```python
from build123d import *

# Parameters (mm, degrees)
SKETCH_1_R      = 1.55
SKETCH_1_W      = 16
SKETCH_1_H      = 6
EXTRUDE_1_DEPTH = 2.2
CHAMFER_1_SIZE  = 3


with BuildPart() as part:
    # 草图1 → 凸台-拉伸1 (new body)
    with BuildSketch(Plane(origin=(0, 0, 0), x_dir=(0, 0, -1), z_dir=(1, 0, 0))):
        with BuildLine():
            Line((-14, -11.5), (14, -11.5))
            Line((14, -11.5), (14, -7.01))
            ThreePointArc((14, -7.01), (12.995, -6.005), (14, -5))
            Line((14, -5), (17, -5))
            Line((17, -5), (17, 5))
            Line((17, 5), (14, 5))
            ThreePointArc((14, 5), (12.995, 6.005), (14, 7.01))
            Line((14, 7.01), (14, 11.5))
            Line((14, 11.5), (6.01, 11.5))
            ThreePointArc((6.01, 11.5), (5.005, 10.495), (4, 11.5))
            Line((4, 11.5), (4, 13.7))
            Line((4, 13.7), (-4, 13.7))
            Line((-4, 13.7), (-4, 11.5))
            ThreePointArc((-4, 11.5), (-5.005, 10.495), (-6.01, 11.5))
            Line((-6.01, 11.5), (-14, 11.5))
            Line((-14, 11.5), (-14, 7.01))
            ThreePointArc((-14, 7.01), (-13.289357685, 6.715642315), (-12.995, 6.005))
            ThreePointArc((-12.995, 6.005), (-13.289357685, 5.294357685), (-14, 5))
            Line((-14, 5), (-17, 5))
            Line((-17, 5), (-17, -5))
            Line((-17, -5), (-14, -5))
            ThreePointArc((-14, -5), (-13.289357685, -5.294357685), (-12.995, -6.005))
            ThreePointArc((-12.995, -6.005), (-13.289357685, -6.715642315), (-14, -7.01))
            Line((-14, -7.01), (-14, -11.5))
        make_face()
        with Locations((0, -7.5)):
            Circle(SKETCH_1_R, mode=Mode.SUBTRACT)
        Rectangle(SKETCH_1_W, SKETCH_1_H, mode=Mode.SUBTRACT)
        with Locations((0, 7.5)):
            Circle(SKETCH_1_R, mode=Mode.SUBTRACT)
    extrude(amount=EXTRUDE_1_DEPTH)

    # 倒角1
    chamfer_1_edges = [part.edges().sort_by_distance(p)[0] for p in [
        (1.1, -11.5, -14),
        (1.1, -11.5, 14),
    ]]
    chamfer(chamfer_1_edges, length=CHAMFER_1_SIZE)


solid = part.part
```
Can you work these out from the model? Positions are in its coordinate system, mm. A direction names the side the tool comes from. Coordinates: 2 decimals unless noted, no trailing zeros. Write each loop counter-clockwise with the first axis right and the second up, starting at its lowest first coordinate (ties: lowest second). Pieces come first, ordered by that corner, then holes. Notation, with made-up numbers: (7.25, -11.5) - (34.25, -11.5) arc R19 ccw to (34.25, -2.5) - close; hole circle Ø1 at (63, 59.5). An arc over 180 degrees is marked (long way). Return JSON: item names as keys, results as strings.
Q1. If we section it at B-B (z = 0): Please give me the cut outline in (x, y), then the cut area to 3 significant figures.
Computed values:
{"outline": "(0, -11.5) - (2.2, -11.5) - (2.2, -9.05) - (0, -9.05) - close; (0, -5.95) - (2.2, -5.95) - (2.2, -3) - (0, -3) - close; (0, 3) - (2.2, 3) - (2.2, 5.95) - (0, 5.95) - close; (0, 9.05) - (2.2, 9.05) - (2.2, 13.7) - (0, 13.7) - close", "area": "28.6 mm2"}
Q2. Please list where these lines run through material, in increasing order: L1, parallel to Y at x = 0.65, z = 0; L2, parallel to Y at x = 1.8, z = 14.5; L3, parallel to Y at x = 0.3, z = 11.5. Write a range as from..to.
Computed values:
{"L1": "y = -11.5..-9.05, -5.95..-3, 3..5.95, 9.05..13.7", "L2": "y = -5..5", "L3": "y = -11..11.5"}
Q3. I'm going to push flat-ended pins straight in: pin 1 Ø0.7 at (x, z) = (1, 8) entering from +Y; pin 2 Ø0.7 at (x, y) = (1.5, 10) entering from +Z; pin 3 Ø1.1 at (x, y) = (1, 12.5) entering from -Z; pin 4 Ø1 at (y, z) = (2, 7) entering from +X. Where does each tip first touch, or does it pass through?
Computed values:
{"pin 1": "stops at y = 11.5", "pin 2": "stops at z = 14", "pin 3": "stops at z = -4", "pin 4": "passes through"}
Q4. If we section it at C-C (z = 7): Please give me the cut outline in (x, y).
Computed values:
{"outline": "(0, -11.5) - (2.2, -11.5) - (2.2, -3) - (0, -3) - close; (0, 3) - (2.2, 3) - (2.2, 11.5) - (0, 11.5) - close"}
Q5. If we section it at A-A (y = 2): Please give me the cut outline in (x, z), then the cut area to 3 significant figures.
Computed values:
{"outline": "(0, -17) - (2.2, -17) - (2.2, -8) - (0, -8) - close; (0, 8) - (2.2, 8) - (2.2, 17) - (0, 17) - close", "area": "39.6 mm2"}
Q6. Thinking about a two-plate mould opening in Y: for faces 5 (the flat face through (1, -3, 0)), 6 (the flat face through (1, 11.5, -10)), 7 (the flat face through (1.1, -10, -12.5)), which applies, +Y half, -Y half, draft (parallel to the pull), parting line (faces both ways), or undercut?
Computed values:
{"face 5": "undercut", "face 6": "+Y half", "face 7": "-Y half"}
Q7. If we section it at D-D (x = 0.7): Count the separate pieces of the cut face and the enclosed holes in it, then the cut area to 3 significant figures.
Computed values:
{"separate pieces": "1", "enclosed holes": "3", "area": "592 mm2"}
Q8. On a 3-axis mill with a long thin cutter (end or side, diameter ignored), from which of +Z, -Z, +X, -X, +Y, -Y can I reach the whole of each face in a straight line? I mean faces 1 (the flat face through (1, -5, 16)), 2 (the flat face through (1, 3, 0)), 3 (the flat face through (1, -8, -14)), 4 (the flat face through (1, 11.5, 10)). Say none if no direction works.
Computed values:
{"face 1": "+Z, +X, -X, -Y", "face 2": "+X, -X", "face 3": "-Z, +X, -X, -Y", "face 4": "+Z, +X, -X, +Y"}
